```python
from build123d import *

# Parameters (mm, degrees)
BASPROSKE_W             = 10
BASPROSKE_H             = 12.25
TOOTHCUT_DEPTH          = 21.003124756
TEETHCUTS_COUNT         = 12
TEETHCUTS_ANGLE         = 330
BORSKE_R                = 4.5
BORE_DEPTH              = 50.0000508
ESQUISSE4_R             = 16.84973796
ENL_V_MAT_EXTRU_2_DEPTH = 2
ESQUISSE5_R             = 5.070841349
BOSS_EXTRU_7_DEPTH      = 8
ESQUISSE6_R             = 4
BOSS_EXTRU_8_DEPTH      = 8.5
ESQUISSE7_W             = 5.65685425
ESQUISSE7_H             = 5.65685425
BOSS_EXTRU_9_DEPTH      = 6
ESQUISSE8_R             = 1.05
ENL_V_MAT_EXTRU_3_DEPTH = 6


with BuildPart() as part:
    # BasProSke → Base-Revolve (revolve)
    with BuildSketch(Plane(origin=(0, 0, 0), x_dir=(1, 0, 0), z_dir=(0, 1, 0)), mode=Mode.PRIVATE) as base_revolve_sk:
        with Locations((5, 6.125)):
            Rectangle(BASPROSKE_W, BASPROSKE_H)
    revolve(base_revolve_sk.sketch.rotate(Axis((-10, 0, 0), (1, 0, 0)), 180), axis=Axis((-10, 0, 0), (1, 0, 0)))

    # TooCutSke → ToothCut (cut, through all)
    with BuildSketch(Plane(origin=(0, 0, 0), x_dir=(0, 0, -1), z_dir=(1, 0, 0))):
        with BuildLine():
            ThreePointArc((0.965128363, 8.255274647), (0, 8.3115), (-0.965128363, 8.255274647))
            ThreePointArc((-0.965128363, 8.255274647), (-1.43628674, 10.346733197), (-2.878284339, 11.933185846))
            ThreePointArc((-2.878284339, 11.933185846), (0, 12.2754), (2.878284339, 11.933185846))
            ThreePointArc((2.878284339, 11.933185846), (1.43628674, 10.346733197), (0.965128363, 8.255274647))
        make_face()
    toothcut = extrude(amount=TOOTHCUT_DEPTH, mode=Mode.SUBTRACT)

    # TeethCuts: ToothCut ×12 about axis
    teethcuts_axis = Axis((-10, 0, 0), (1, 0, 0))
    for i in range(1, TEETHCUTS_COUNT):
        add(toothcut.rotate(teethcuts_axis, i * TEETHCUTS_ANGLE / (TEETHCUTS_COUNT - 1)), mode=Mode.SUBTRACT)

    # BorSke → Bore (cut, symmetric)
    with BuildSketch(Plane(origin=(0, 0, 0), x_dir=(0, 0, -1), z_dir=(1, 0, 0))):
        with Locations(Location((0, 0, 0), (0, 0, 180))):
            Circle(BORSKE_R)
    extrude(amount=BORE_DEPTH, both=True, mode=Mode.SUBTRACT)

    # Esquisse4 → Enlèv. mat.-Extru.2 (cut)
    with BuildSketch(Plane.ZY):
        Circle(ESQUISSE4_R)
    extrude(amount=-ENL_V_MAT_EXTRU_2_DEPTH, mode=Mode.SUBTRACT)

    # Esquisse5 → Boss.-Extru.7 (add)
    with BuildSketch(Plane.ZY.offset(-2)):
        Circle(ESQUISSE5_R)
    extrude(amount=-BOSS_EXTRU_7_DEPTH)

    # Esquisse6 → Boss.-Extru.8 (add)
    with BuildSketch(Plane.ZY.offset(-2)):
        Circle(ESQUISSE6_R)
    extrude(amount=BOSS_EXTRU_8_DEPTH)

    # Esquisse7 → Boss.-Extru.9 (add)
    with BuildSketch(Plane.ZY.offset(6.5)):
        Rectangle(ESQUISSE7_W, ESQUISSE7_H)
    extrude(amount=BOSS_EXTRU_9_DEPTH)

    # Esquisse8 → Enlèv. mat.-Extru.3 (cut)
    with BuildSketch(Plane(origin=(0, 0, -2.828427125), x_dir=(-1, 0, 0), z_dir=(0, 0, -1))):
        with Locations((9.5, 0)):
            Circle(ESQUISSE8_R)
    extrude(amount=-ENL_V_MAT_EXTRU_3_DEPTH, mode=Mode.SUBTRACT)


solid = part.part
```
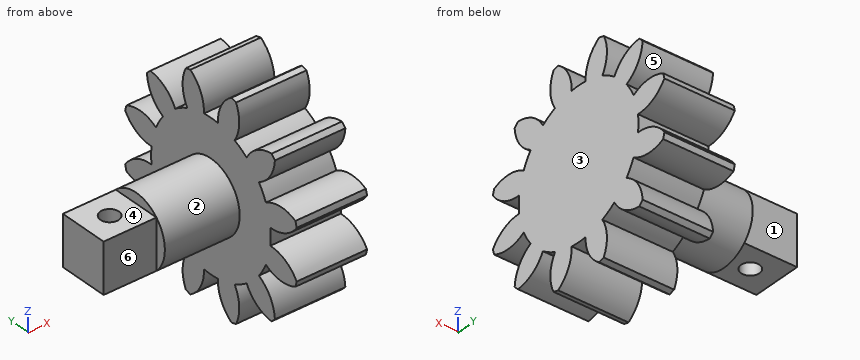
Source: CAD feature listing. Evaluate the final solid. Frame: model axes, mm. Face numbers are marked on the shaded views. A direction names the side the tool comes from. Coordinates: 2 decimals unless noted, no trailing zeros. Loops run counter-clockwise (first coordinate to the right, second up) from the corner with the lowest first, then second, coordinate; pieces in that order, holes last. Notation, with made-up numbers: M -13.5,-22.75 L 26.5,-22.75 A22 cw 26.5,0.25 Z; hole C 20.25,-29.75 d6. An arc over 180 degrees is marked long. Put each result on its own line as item: value. Start each with the question number.
1) Cut plane D-D on x = -7. Return the cut outline in (y, z), then the cut area to 3 significant figures.
2) Cut plane B-B on z = 0. Return the cut outline in (x, y), then the cut area to 3 significant figures.
3) Contact query for flat-ended pins moving along their axis: pin 1 Ø1 at (x, z) = (2.5, 3.5) entering from -Y; pin 2 Ø1 at (x, z) = (-1.5, 2) entering from -Y; pin 3 Ø6 at (x, y) = (-9, -1) entering from -Z. Output: stop coordinate, or through.
4) Cut plane C-C on y = 0. Return the cut outline in (x, z).
5) Ray query, L1, parallel to Y at x = -9.5, z = -0.2; L2, parallel to Z at x = 8, y = -6.75; L3, parallel to X at y = 8.5, z = -3.25. Return the intervals inside material, ascending. Write a range as from..to.
6) Cut plane A-A on x = -9.5. Return the cut outline in (y, z).
7) Pull-direction query (Z, two-part tool) for the marked faces 4, 5 and 6; classes: pulls with the +Z half, pulls with the -Z half, needs draft (parallel to the pull), parting line crosses it, or undercut.
8) Reachability of the marked faces 1, 2 and 3 from +Z, -Z, +X, -X, +Y, -Y: full face, straight path, thin tool, end or side. Return the list, or none.
The answers:
1. outline: M -2.83,-2.83 L 2.83,-2.83 L 2.83,2.83 L -2.83,2.83 Z
1. area: 32.0 mm²
2. outline: M -12.5,-2.83 L -6.5,-2.83 L -6.5,-4 L 2,-4 L 2,-8.31 L 10,-8.31 L 10,8.31 L 2,8.31 L 2,4 L -6.5,4 L -6.5,2.83 L -12.5,2.83 Z; hole C -9.5,0 d2.1
2. area: 231 mm²
3. pin 1: stops at y = -11.88
3. pin 2: stops at y = -3.71
3. pin 3: stops at z = -4
4. outline: M -12.5,-2.83 L -10.55,-2.83 L -10.55,2.83 L -12.5,2.83 Z; M -8.45,-2.83 L -6.5,-2.83 L -6.5,-4 L 2,-4 L 2,-8.31 L 10,-8.31 L 10,8.31 L 2,8.31 L 2,4 L -6.5,4 L -6.5,2.83 L -8.45,2.83 Z
5. L1: y = -2.83..-1.05, 1.05..2.83
5. L2: z = -8.43..-5.01, -4.85..4.85, 5.01..8.43
5. L3: x = 2..10
6. outline: M -2.83,-2.83 L -1.05,-2.83 L -1.05,2.83 L -2.83,2.83 Z; M 1.05,-2.83 L 2.83,-2.83 L 2.83,2.83 L 1.05,2.83 Z
7. face 4: pulls with the +Z half
7. face 5: undercut
7. face 6: needs draft
8. face 1: +Z, -Z, -X, +Y
8. face 2: -X
8. face 3: +Z, -Z, +X, +Y, -Y
